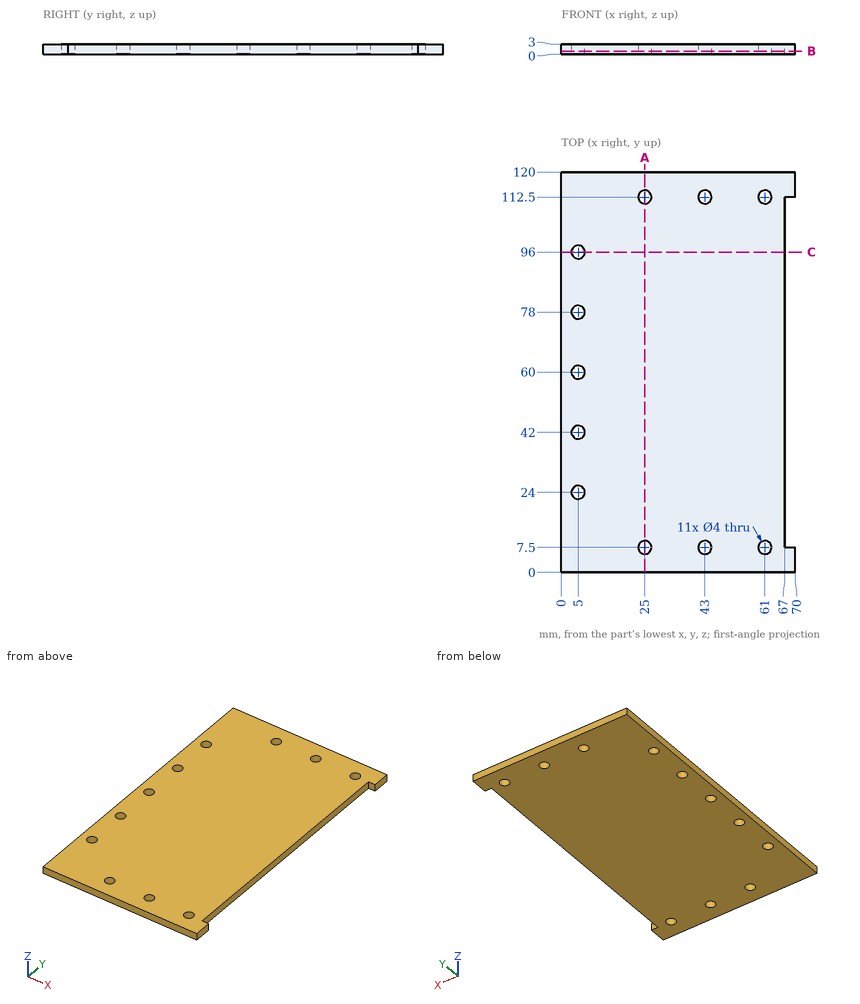
For this review, use the dimensioned drawing (mm, ordinates from the lowest corner) and the shaded views. Coordinates: 2 decimals unless noted, no trailing zeros. Loops run counter-clockwise (first coordinate to the right, second up) from the corner with the lowest first, then second, coordinate; pieces in that order, holes last. Notation, with made-up numbers: (-6, 12.5) -> (13, 12.5) arc R20 cw to (13, 21.5) -> close; hole circle Ø3 at (-37, 47). An arc over 180 degrees is marked (long way). Use a Markdown table: item, result. Add a question column.
Item 1: We need section B-B, the plane z = 0.9. Count the separate pieces of the cut face and the enclosed holes in it, and give its area (3 significant figures).
Item 2: Wall thickness on L1, parallel to Y at x = 5, z = 2.3; L2, parallel to Y at x = 43, z = 2.05; L3, parallel to Y at x = 3.5, z = 1.4: over which ranges is each line inside the solid? List them lowest first. Write a range as from..to.
Item 3: We need section C-C, the plane y = 96. Write out the cut boundary in (x, z), and give its area (3 significant figures).
Item 4: We need section A-A, the plane x = 25. Write out the cut boundary in (y, z), and give its area (3 significant figures).
Numbers:
| question | item | result |
|---|---|---|
| 1 | separate pieces | 1 |
| 1 | enclosed holes | 11 |
| 1 | area | 7,950 mm^2 |
| 2 | L1 | y = 0..22, 26..40, 44..58, 62..76, 80..94, 98..120 |
| 2 | L2 | y = 0..5.5, 9.5..110.5, 114.5..120 |
| 2 | L3 | y = 0..22.68, 25.32..40.68, 43.32..58.68, 61.32..76.68, 79.32..94.68, 97.32..120 |
| 3 | outline | (0, 0) -> (3, 0) -> (3, 3) -> (0, 3) -> close; (7, 0) -> (67, 0) -> (67, 3) -> (7, 3) -> close |
| 3 | area | 189 mm^2 |
| 4 | outline | (0, 0) -> (5.5, 0) -> (5.5, 3) -> (0, 3) -> close; (9.5, 0) -> (110.5, 0) -> (110.5, 3) -> (9.5, 3) -> close; (114.5, 0) -> (120, 0) -> (120, 3) -> (114.5, 3) -> close |
| 4 | area | 336 mm^2 |
